from build123d import *

# Parameters (mm, degrees)
BOSS_EXTRU_1_DEPTH                    = 8
ESQUISSE2_W                           = 8
ESQUISSE2_H                           = 20
BOSS_EXTRU_2_DEPTH                    = 100
BOSS_EXTRU_2_DEPTH_BACK               = 5
ESQUISSE3_R                           = 12
BOSS_EXTRU_3_DEPTH                    = 8
ESQUISSE4_R                           = 12
BOSS_EXTRU_4_DEPTH                    = 8
DIAM_TRE_DU_PER_AGE_4_1_4_1_1_D       = 4.1
DIAM_TRE_DU_PER_AGE_15_5_15_5_1_D     = 15.5
DIAM_TRE_DU_PER_AGE_15_5_15_5_1_DEPTH = 16
D_GAGEMENT_M2_51_D                    = 2.85
D_GAGEMENT_M2_51_DEPTH                = 10
CONG_1_R                              = 5


with BuildPart() as part:
    # Esquisse1 → Boss.-Extru.1 (new body)
    with BuildSketch(Plane.XY.offset(8)):
        with BuildLine():
            Line((-12, 44.000000179), (-12, 0))
            ThreePointArc((-12, 0), (0, -12), (12, 0))
            Line((12, 0), (12, 12))
            Line((12, 12), (0, 12))
            Line((0, 12), (0, 32))
            Line((0, 32), (12, 32))
            Line((12, 32), (12, 44.000000179))
            ThreePointArc((12, 44.000000179), (0, 56.000000179), (-12, 44.000000179))
        make_face()
    extrude(amount=-BOSS_EXTRU_1_DEPTH)

    # Esquisse2 → Boss.-Extru.2 (add, two sides)
    with BuildSketch(Plane.ZY.offset(12)) as boss_extru_2_sk:
        with Locations((4, 2)):
            Rectangle(ESQUISSE2_W, ESQUISSE2_H)
    extrude(amount=BOSS_EXTRU_2_DEPTH)
    extrude(boss_extru_2_sk.sketch, amount=-BOSS_EXTRU_2_DEPTH_BACK)

    # Esquisse3 → Boss.-Extru.3 (add)
    with BuildSketch(Plane.XY.offset(8)):
        with Locations((0, 44)):
            Circle(ESQUISSE3_R)
    extrude(amount=BOSS_EXTRU_3_DEPTH)

    # Esquisse4 → Boss.-Extru.4 (add)
    with BuildSketch(Plane.XY.offset(8)):
        Circle(ESQUISSE4_R)
    extrude(amount=BOSS_EXTRU_4_DEPTH)

    # Diamètre du perçage Ø4.1 (4.1)1 (through all)
    with Locations(Plane.XY.offset(8)):
        with Locations((-39.923806844, 2), (-92, 2)):
            Hole(DIAM_TRE_DU_PER_AGE_4_1_4_1_1_D / 2)

    # Diamètre du perçage Ø15.5 (15.5)1
    with Locations(Plane.XY.offset(16)):
        with Locations((0, 44), (0, 0)):
            Hole(DIAM_TRE_DU_PER_AGE_15_5_15_5_1_D / 2, depth=DIAM_TRE_DU_PER_AGE_15_5_15_5_1_DEPTH)

    # Dégagement M2.51
    with Locations(Plane(origin=(0, 0, 0), x_dir=(0, 0, -1), z_dir=(1, 0, 0))):
        with Locations((-4.029990313, 22)):
            Hole(D_GAGEMENT_M2_51_D / 2, depth=D_GAGEMENT_M2_51_DEPTH)

    # Congé1
    cong_1_edges = [part.edges().sort_by_distance(p)[0] for p in [
        (-12, 12, 4),
        (-8.94427191, -8, 4),
    ]]
    fillet(cong_1_edges, radius=CONG_1_R)


solid = part.part
Here's how the part is built. I have some questions about the finished solid (model axes, mm). A direction names the side the tool comes from. Round coordinates to 2 decimals unless told otherwise and drop trailing zeros. Loops run counter-clockwise (first coordinate to the right, second up) from the corner with the lowest first, then second, coordinate; pieces in that order, holes last.
1. Which directions (+Z, -Z, +X, -X, +Y, -Y) give clear straight access to the entire face, cutting with the end or side of a thin tool? Please do faces 1 (the face through (5.537, -10.646, 9.666)), 2 (the face through (-64, 12, 4)), 3 (the face through (9, 34, 8)), 4 (the face through (6, 12, 4)).
Answer list:
face 1: +Z
face 2: +Z, -Z, -X, +Y
face 3: +Z, +X
face 4: +Z, -Z, +X
2. We'd pull the mould along Z, two halves only. Please class faces 5 (the face through (-10, 22, 4)), 6 (the face through (-5.07, 20.61, 3.72)), 7 (the face through (-12, 31, 4)), 8 (the face through (-57, 5, 8)): +Z half, -Z half, draft (parallel to the pull), parting line (faces both ways), or undercut.
Answer list:
face 5: undercut
face 6: undercut
face 7: draft
face 8: +Z half
3. If we section it at A-A on z = 6.75: Write out the boundary of the cut face in (x, y).
Answer list:
outline: (-112, -8) - (-10.95, -8) arc R5 cw to (-7.73, -9.18) arc R12 ccw to (12, 0) - (12, 12) - (0, 12) - (0, 32) - (12, 32) - (12, 44) arc R12 ccw to (-12, 44) - (-12, 17) arc R5 cw to (-17, 12) - (-112, 12) - close; hole circle Ø4.1 at (-92, 2); hole circle Ø4.1 at (-39.92, 2); hole circle Ø15.5 at (0, 0); hole circle Ø15.5 at (0, 44)
4. If we section it at C-C on x = -99.5: Write out the boundary of the cut face in (y, z), plus the area to 3 significant figures.
Answer list:
outline: (-8, 0) - (12, 0) - (12, 8) - (-8, 8) - close
area: 160 mm2
5. For P1, Ø4, axis at x = 8, z = 5, coming from the +Y side; P2, Ø2.5, axis at x = -39.5, z = 5, coming from the -Y side; P3, Ø4, axis at y = 34, z = 5, coming from the -X side; P4, Ø9.5, axis at x = 0, y = 44, coming from the -Z side, each with a flat end and sliding along its axis, tell me the tip position at first contact or that it passes through.
Answer list:
P1: stops at y = 54.39
P2: stops at y = -8
P3: stops at x = -12
P4: passes through
6. If I drill on line 1 along Y through (x, z) = (0, 10.25); line 2 along Y through (x, z) = (-92, 2.5); line 3 along X through (y, z) = (45.5, 4.5), over which ranges is the centre line in solid material (lowest first)?
Answer list:
line 1: y = -12 to -7.75, 7.75 to 12, 32 to 36.25, 51.75 to 56
line 2: y = -8 to -0.05, 4.05 to 12
line 3: x = -11.91 to -7.6, 7.6 to 11.91
7. If we section it at B-B on y = 45.5: Write out the boundary of the cut face in (x, z).
Answer list:
outline: (-11.91, 0) - (-7.6, 0) - (-7.6, 16) - (-11.91, 16) - close; (7.6, 0) - (11.91, 0) - (11.91, 16) - (7.6, 16) - close
8. If we section it at D-D on y = 35: Write out the boundary of the cut face in (x, z), plus the area to 3 significant figures.
Answer list:
outline: (-12, 0) - (12, 0) - (12, 8) - (7.94, 8) - (7.94, 16) - (-7.94, 16) - (-7.94, 8) - (-12, 8) - close
area: 319 mm2
